from build123d import *

# Parameters (mm, degrees)
CYLINDER860_R          = 1.5
CYLINDER860_DEPTH      = 60
CYLINDER859_R          = 1.5
CYLINDER859_DEPTH      = 60
BOX336_W               = 20
BOX336_H               = 40
BOX336_DEPTH           = 60
BOX336_PLACEMENT_ANGLE = 22
BOX410_W               = 20
BOX410_H               = 40
BOX410_DEPTH           = 60
BOX410_PLACEMENT_ANGLE = 22
BOX335_W               = 60
BOX335_H               = 40
BOX335_DEPTH           = 60
TUBE037_R              = 20.5
TUBE037_R_2            = 12
TUBE037_DEPTH          = 27
CUT470_PLACEMENT_ANGLE = 210


with BuildPart() as obj1:
    # Cylinder860 → Cylinder860 (new body)
    with BuildSketch(Plane(origin=(-3.5, 16, 0), x_dir=(1, 0, 0), z_dir=(0, 0, 1))):
        Circle(CYLINDER860_R)
    extrude(amount=CYLINDER860_DEPTH)


with BuildPart() as compound565:
    # Cylinder859 → Cylinder859 (new body)
    with BuildSketch(Plane(origin=(3.5, 16, 0), x_dir=(1, 0, 0), z_dir=(0, 0, 1))):
        Circle(CYLINDER859_R)
    extrude(amount=CYLINDER859_DEPTH)

    # Compound565: union obj1
    add(obj1.part)


with BuildPart() as krychle336:
    # Box336 → Box336 (new body)
    with BuildSketch(Plane.XY):
        with Locations((10, 20)):
            Rectangle(BOX336_W, BOX336_H)
    extrude(amount=BOX336_DEPTH)


with BuildPart() as krychle336_1:
    # Box336 placement: moved
    add(krychle336.part.rotate(Axis((0, 0, 0), (0, 0, -1)), BOX336_PLACEMENT_ANGLE))


with BuildPart() as krychle410:
    # Box410 → Box410 (new body)
    with BuildSketch(Plane.XY):
        with Locations((10, 20)):
            Rectangle(BOX410_W, BOX410_H)
    extrude(amount=BOX410_DEPTH)


with BuildPart() as krychle410_1:
    # Box410 placement: moved
    add(krychle410.part.moved(Location((-19.32, -5.18, 0))).rotate(Axis((-19.32, -5.18, 0), (0, 0, 1)), BOX410_PLACEMENT_ANGLE))


with BuildPart() as krychle335:
    # Box335 → Box335 (new body)
    with BuildSketch(Plane(origin=(-30, -35, 0), x_dir=(1, 0, 0), z_dir=(0, 0, 1))):
        with Locations((30, 20)):
            Rectangle(BOX335_W, BOX335_H)
    extrude(amount=BOX335_DEPTH)


with BuildPart() as cut470:
    # Tube037 → Tube037 (new body)
    with BuildSketch(Plane.XY.offset(23)):
        Circle(TUBE037_R)
        Circle(TUBE037_R_2, mode=Mode.SUBTRACT)
    extrude(amount=TUBE037_DEPTH)

    # Cut355: cut Krychle335
    add(krychle335.part, mode=Mode.SUBTRACT)

    # Cut357: cut Krychle410
    add(krychle410_1.part, mode=Mode.SUBTRACT)

    # Cut358: cut Krychle336
    add(krychle336_1.part, mode=Mode.SUBTRACT)

    # Cut470: cut Compound565
    add(compound565.part, mode=Mode.SUBTRACT)


with BuildPart() as cut470_1:
    # Cut470 placement: moved
    add(cut470.part.rotate(Axis((0, 0, 0), (0, 0, 1)), CUT470_PLACEMENT_ANGLE))


solid = cut470_1.part
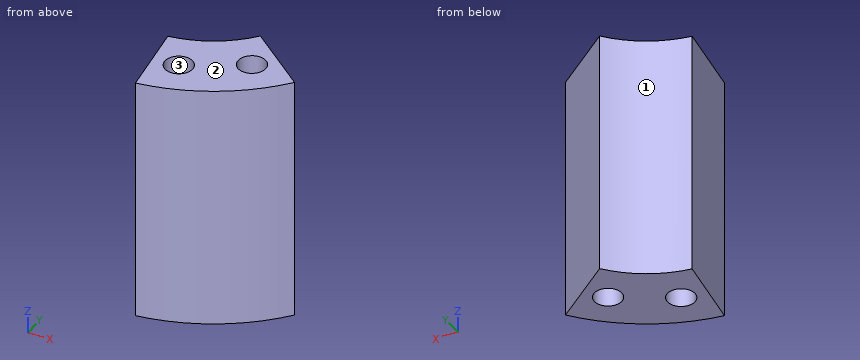
Part model, mm, in its own coordinate system. Face numbers are marked on the shaded views. Give positions to 0.01 mm unless a question says otherwise; leave off trailing zeros. Write each loop counter-clockwise with the first axis right and the second up, starting at its lowest first coordinate (ties: lowest second). Pieces come first, ordered by that corner, then holes.
1) Two-plate mould, pull along Y, no slides. Class the marked faces 1, 2 and 3: released by +Y, released by -Y, zero draft, split by the parting line, or undercut.
Resolved:
face 1: released by +Y
face 2: zero draft
face 3: undercut
2) Pin check, flat tips, straight feed: pin 1 (1 mm diameter, centred on y = -14.5, z = 39, fed in from +X) (3 decimals); pin 2 (8 mm diameter, centred on x = 3, z = 41, fed in from -Y); pin 3 (1.5 mm diameter, centred on y = -15, z = 29, fed in from -X). Stop position of each tip, or through.
Resolved:
pin 1: stops at x = 14.975
pin 2: stops at y = -20.3
pin 3: stops at x = 2
3) Probe L1, parallel to X at y = -14.75, z = 43.25; L2, parallel to Y at x = 12.25, z = 35.25; L3, parallel to X at y = -11, z = 36. List the from-to ranges inside material, lowest first.
Resolved:
L1: x = 2.07 to 3.74, 6.2 to 14.24
L2: y = -16.44 to -12.98, -11.23 to -9.76
L3: x = 4.8 to 10.02, 12.04 to 13.84
4) Cut at B-B on x = 10.5. Write the cut outline in (y, z).
Resolved:
outline: (-17.61, 23) - (-13.51, 23) - (-13.51, 50) - (-17.61, 50) - close; (-10.7, 23) - (-8.39, 23) - (-8.39, 50) - (-10.7, 50) - close
5) Cut at D-D on x = 14. Write the cut outline in (y, z), then the cut area to 3 significant figures.
Resolved:
outline: (-14.97, 23) - (-11.12, 23) - (-11.12, 50) - (-14.97, 50) - close
area: 104 mm2
6) Cut at A-A on y = -11.5. Write the cut outline in (x, z), then the cut area to 3 significant figures.
Resolved:
outline: (3.43, 23) - (9.66, 23) - (9.66, 50) - (3.43, 50) - close; (12.4, 23) - (14.48, 23) - (14.48, 50) - (12.4, 50) - close
area: 224 mm2
7) Cut at C-C on z = 37.75. Write the cut outline in (x, y).
Resolved:
outline: (1.67, -11.88) - (2.85, -20.3) arc R20.5 ccw to (16.06, -12.74) - (9.37, -7.5) arc R12 cw to start; hole circle Ø3 at (4.97, -15.61); hole circle Ø3 at (11.03, -12.11)
